Autodesk Fusion 360 part; units mm, degrees
sketch "Sketch1" plane through (0, 0, 0) normal (0, 0, 1) x (1, 0, 0)
  line L0 (-7.5, 2.5) -> (46.7, 2.5)
  line L1 (46.7, 2.5) -> (46.7, -11.6)
  line L2 (46.7, -11.6) -> (-7.5, -11.6)
  line L3 (-7.5, -11.6) -> (-7.5, 2.5)
  line L4 (46.7, -11.6) -> (-7.5, -11.6)
  line L5 (-7.5, -11.6) -> (-7.5, -6.7)
  line L6 (-7.5, -6.7) -> (46.7, -6.7)
  line L7 (46.7, -6.7) -> (46.7, -11.6)
  dimension "d1" = 54.2
  dimension "d2" = 14.1
  dimension "d3" = 4.9
extrude "Extrude1" add sketch "Sketch1" along normal blind 5 contours L0 L1 L3 L6
extrude "Extrude2" add sketch "Sketch1" along normal blind 1.35 contours L1 L2 L3 L4 L5 L6 L7
sketch "Sketch2" plane through (0, 0, 5) normal (0, 0, 1) x (-1, 0, 0)
  line L0 (7.5, -2.5) -> (7.5, 6.7)
  line L1 (7.5, 6.7) -> (-46.7, 6.7)
  line L2 (-46.7, 6.7) -> (-46.7, -2.5)
  line L3 (-46.7, -2.5) -> (7.5, -2.5)
  line L4 (-19.6, -2.5) -> (-46.7, -2.5)
  line L5 (-46.7, -2.5) -> (-46.7, 6.7)
  line L6 (-46.7, 6.7) -> (-19.6, 6.7)
  line L7 (-46.7, 2.1) -> (-46.7, 6.7)
  line L8 (-46.7, 6.7) -> (7.5, 6.7)
  line L9 (7.5, 6.7) -> (7.5, 2.1)
  circle A0 centre (-19.6, 2.1) radius 1.7
  line L10 (-36.7, 6.7) -> (-46.7, 6.7)
  line L11 (-46.7, 6.7) -> (-46.7, 2.1)
  line L12 (-2.5, 6.7) -> (7.5, 6.7)
  line L13 (7.5, 6.7) -> (7.5, 2.1)
  circle A1 centre (-2.5, 2.1) radius 1
  circle A2 centre (-36.7, 2.1) radius 1
  dimension "d8" = 3.4
  dimension "d9" = 10
  dimension "d10" = 10
  dimension "d11" = 2
  dimension "d12" = 2
extrude "Extrude3" cut sketch "Sketch2" against normal blind 18 contours A0
extrude "Extrude4" add sketch "Sketch2" along normal blind 2.9 contours A1 | A2
sketch "Sketch3" plane through (-7.5, 0, 0) normal (-1, 0, 0) x (0, -1, 0)
  line L0 (-2.5, 0) -> (11.6, 0)
  line L1 (11.6, 0) -> (11.6, 1.35)
  line L2 (11.6, 1.35) -> (6.7, 1.35)
  line L3 (6.7, 1.35) -> (6.7, 5)
  line L4 (6.7, 5) -> (-2.5, 5)
  line L5 (-2.5, 5) -> (-2.5, 0)
  line L6 (-2.5, 5) -> (2.5, 5)
  line L7 (2.5, 5) -> (2.5, 0)
  line L8 (2.5, 0) -> (-2.5, 0)
  line L9 (-2.5, 0) -> (-2.5, 5)
  circle A0 centre (2.5, 5) radius 5
  dimension "d17" = 5
extrude "Extrude5" cut sketch "Sketch3" against normal blind 63 contours L0 L5 L8 L9 A0
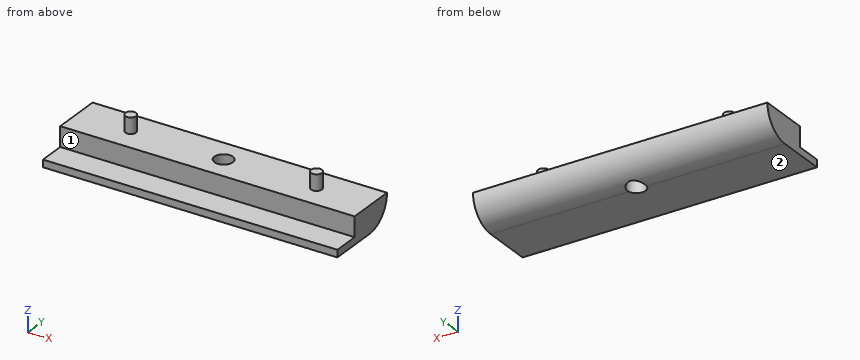
Work out the finished part from the listing and answer in its coordinate system (mm). Face numbers are marked on the shaded views. A direction names the side the tool comes from. Give positions to 0.01 mm unless a question says otherwise; leave off trailing zeros. Loops run counter-clockwise (first coordinate to the right, second up) from the corner with the lowest first, then second, coordinate; pieces in that order, holes last. Notation, with made-up numbers: (42.25, 30.25) -> (48.25, 30.25) arc R19 ccw to (48.25, 45.25) -> close; hole circle Ø4 at (87.5, 21). An arc over 180 degrees is marked (long way). Use a Markdown table: item, result. Add a question column.
1. For the marked faces 1 and 2, determine the directions among +Z, -Z, +X, -X, +Y, -Y from which every point of the face is accessible in a straight line to the end or side of a thin tool.
2. Section C-C on x = 19.6 is taken. Determine the outline of the cut face in (y, z), and give its area (3 significant figures).
3. Section B-B on z = 6.75 is taken. Determine the outline of the cut face in (x, y).
4. Section D-D on z = 3.25 is taken. Determine the outline of the cut face in (x, y), and give its area (3 significant figures).
5. Flat-ended cylindrical pins translate along their axes: pin 1 Ø4 at (x, y) = (6.5, 0) entering from -Z; pin 2 Ø1.8 at (x, z) = (24.5, 2.5) entering from -Y; pin 3 Ø2.5 at (x, y) = (23, -9.5) entering from +Z. Find the tip coordinate at first contact, or state that the pin passes through.
6. Find the intervals of material crossed by probe 1 along X at (y, z) = (-2.1, 3.35); probe 2 along Z at (x, y) = (42.5, -7); probe 3 along Z at (x, y) = (1, -6), in increasing order.
7. Section A-A on x = 36.7 is taken. Determine the outline of the cut face in (y, z).
Results below:
| question | item | result |
|---|---|---|
| 1 | face 1 | +Z, +X, -X, -Y |
| 1 | face 2 | -Z, +X, -X, +Y, -Y |
| 2 | outline | (-11.6, 0) -> (-3.8, 0) -> (-3.8, 5) -> (-6.7, 5) -> (-6.7, 1.35) -> (-11.6, 1.35) -> close; (-0.4, 0.46) arc R5 ccw to (2.5, 5) -> (-0.4, 5) -> close |
| 2 | area | 30.6 mm^2 |
| 3 | outline | circle Ø2 at (2.5, -2.1); circle Ø2 at (36.7, -2.1) |
| 4 | outline | (-7.5, -6.7) -> (46.7, -6.7) -> (46.7, 2.18) -> (-7.5, 2.18) -> close; hole circle Ø3.4 at (19.6, -2.1) |
| 4 | area | 472 mm^2 |
| 5 | pin 1 | stops at z = 0.03 |
| 5 | pin 2 | stops at y = -6.7 |
| 5 | pin 3 | stops at z = 1.35 |
| 6 | probe 1 | x = -7.5 to 17.9, 21.3 to 46.7 |
| 6 | probe 2 | z = 0 to 1.35 |
| 6 | probe 3 | z = 0 to 5 |
| 7 | outline | (-11.6, 0) -> (-2.5, 0) arc R5 ccw to (2.5, 5) -> (-1.1, 5) -> (-1.1, 7.9) -> (-3.1, 7.9) -> (-3.1, 5) -> (-6.7, 5) -> (-6.7, 1.35) -> (-11.6, 1.35) -> close |
